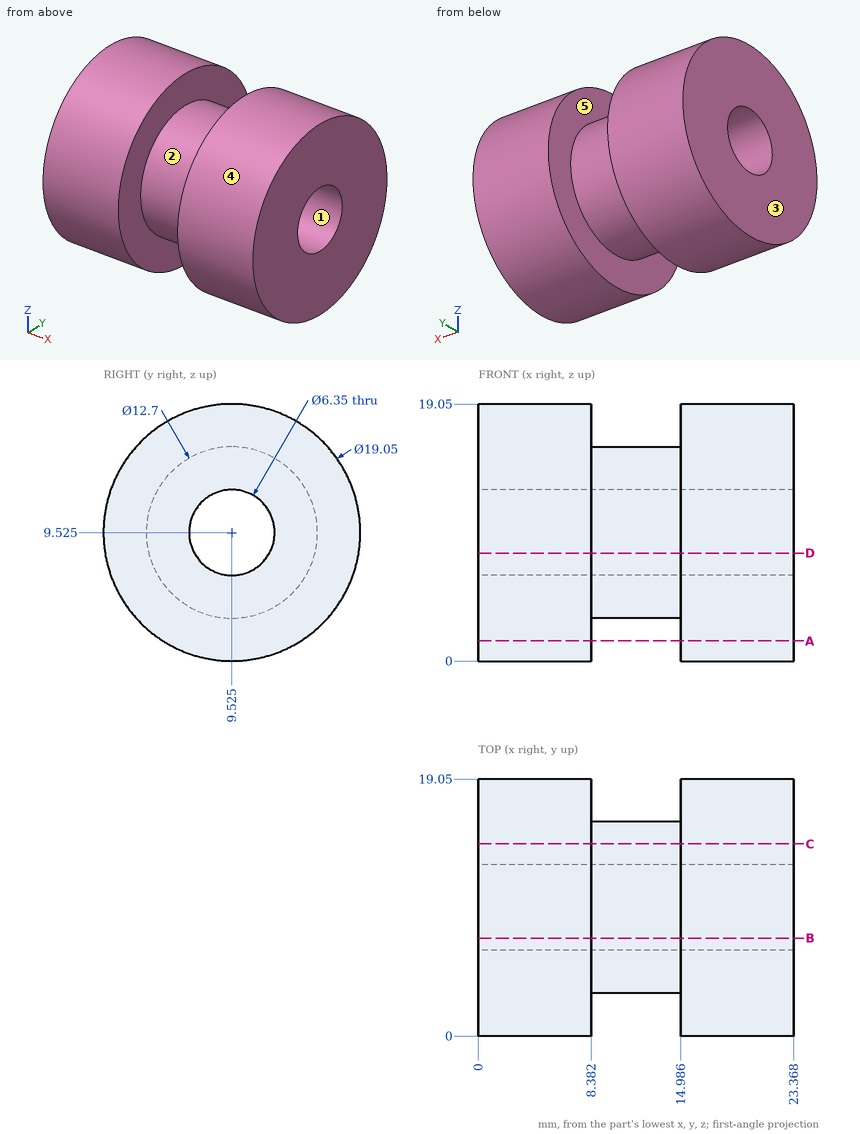
Job drawing, mm, ordinate dimensions from the low corner. One solid piece. A direction names the side the tool comes from. Round coordinates to 2 decimals unless told otherwise and drop trailing zeros. Loops run counter-clockwise (first coordinate to the right, second up) from the corner with the lowest first, then second, coordinate; pieces in that order, holes last. Notation, with made-up numbers: (-11.5, 5) -> (42.5, 5) arc R15 cw to (42.5, 14) -> close; hole circle Ø11 at (70.5, 79). An arc over 180 degrees is marked (long way). Use a Markdown table: item, result.
1) Cut at D-D, the plane z = 8. List the corners of the cut face in (x, y).
The answers:
| item | result |
|---|---|
| outline | (0, 0.12) -> (8.38, 0.12) -> (8.38, 3.36) -> (14.99, 3.36) -> (14.99, 0.12) -> (23.37, 0.12) -> (23.37, 6.74) -> (0, 6.74) -> close; (0, 12.31) -> (23.37, 12.31) -> (23.37, 18.93) -> (14.99, 18.93) -> (14.99, 15.69) -> (8.38, 15.69) -> (8.38, 18.93) -> (0, 18.93) -> close |
2) Pull direction X, two halves, no side cores. Call the marked faces 3, 4 and 5: pulls with the +X half, pulls with the -X half, needs draft (parallel to the pull), parting line crosses it, or undercut.
The answers:
| item | result |
|---|---|
| face 3 | pulls with the -X half |
| face 4 | needs draft |
| face 5 | undercut |
3) Cut at B-B, the plane y = 7.25. List the corners of the cut face in (x, z), and give its area (3 significant figures).
The answers:
| item | result |
|---|---|
| outline | (0, 0.28) -> (8.38, 0.28) -> (8.38, 3.6) -> (14.99, 3.6) -> (14.99, 0.28) -> (23.37, 0.28) -> (23.37, 7.31) -> (0, 7.31) -> close; (0, 11.74) -> (23.37, 11.74) -> (23.37, 18.77) -> (14.99, 18.77) -> (14.99, 15.45) -> (8.38, 15.45) -> (8.38, 18.77) -> (0, 18.77) -> close |
| area | 285 mm2 |
4) Cut at C-C, the plane y = 14.25. List the corners of the cut face in (x, z), and give its area (3 significant figures).
The answers:
| item | result |
|---|---|
| outline | (0, 1.25) -> (8.38, 1.25) -> (8.38, 5.28) -> (14.99, 5.28) -> (14.99, 1.25) -> (23.37, 1.25) -> (23.37, 17.8) -> (14.99, 17.8) -> (14.99, 13.77) -> (8.38, 13.77) -> (8.38, 17.8) -> (0, 17.8) -> close |
| area | 333 mm2 |
5) Cut at A-A, the plane z = 1.5. List the corners of the cut face in (x, y), and give its area (3 significant figures).
The answers:
| item | result |
|---|---|
| outline | (0, 4.39) -> (8.38, 4.39) -> (8.38, 14.66) -> (0, 14.66) -> close; (14.99, 4.39) -> (23.37, 4.39) -> (23.37, 14.66) -> (14.99, 14.66) -> close |
| area | 172 mm2 |
6) Tool access for the marked faces 1 and 2: list every direction of +Z, -Z, +X, -X, +Y, -Y with a clear straight run to the whole face (end or side of a thin tool).
The answers:
| item | result |
|---|---|
| face 1 | +X, -X |
| face 2 | none |
7) Probe line 1 (X direction, y = 15, z = 15); line 2 (Y direction, x = 4, z = 8.75); line 3 (Z direction, x = 21.75, y = 9). List the from-to ranges inside material, lowest first. Write a range as [from, to].
The answers:
| item | result |
|---|---|
| line 1 | x = [0, 8.38], [14.99, 23.37] |
| line 2 | y = [0.03, 6.45], [12.6, 19.02] |
| line 3 | z = [0.01, 6.39], [12.66, 19.04] |
8) Drop flat-ended pins along their axis: pin 1 Ø1 at (x, y) = (13, 5.5) entering from +Z; pin 2 Ø1.5 at (x, y) = (4.5, 15.5) entering from +Z; pin 3 Ø6 at (x, y) = (14.5, 6) entering from -Z. Give the stop position or say it passes through.
The answers:
| item | result |
|---|---|
| pin 1 | stops at z = 14.81 |
| pin 2 | stops at z = 17.49 |
| pin 3 | stops at z = 0.02 |
